Here's how the part is built. I have some questions about the finished solid (model axes, mm). Round coordinates to 2 decimals unless told otherwise and drop trailing zeros. Order: outer loops, then holes, each group sorted by start corner. A loop starts at its lowest first (then second) coordinate and runs counter-clockwise, first axis right, second up. Notation, with made-up numbers: (-18.75, 20.5) -> (-6.75, 20.5) arc R15 cw to (-6.75, 32.5) -> close; hole circle Ø2 at (74, -25). An arc over 180 degrees is marked (long way). Use a Markdown table: item, result. Add a question column.
(1) I want a section at A-A, the plane y = 12.7. Please give me the cut outline in (x, z).
(2) If I drill on probe 1 along Y at (x, z) = (0, 0.5); probe 2 along Y at (x, z) = (-12, 0.6); probe 3 along X at (y, z) = (65, 1.3), over which ranges is the centre line in solid material (lowest first)?
(3) I want a section at C-C, the plane z = 0. Please give me the cut outline in (x, y), then the cut area to 3 significant figures.
(4) I want a section at B-B, the plane x = -10. Please give me the cut outline in (y, z), then the cut area to 3 significant figures.
(5) I'm going to push flat-ended pins straight in: P1, Ø1.6, axis at x = 0.5, z = -1, coming from the +Y side; P2, Ø1, axis at y = 121.5, z = 1, coming from the -X side; P3, Ø1, axis at x = -59.5, z = 1, coming from the +Y side. Where does each tip first touch, or does it pass through?
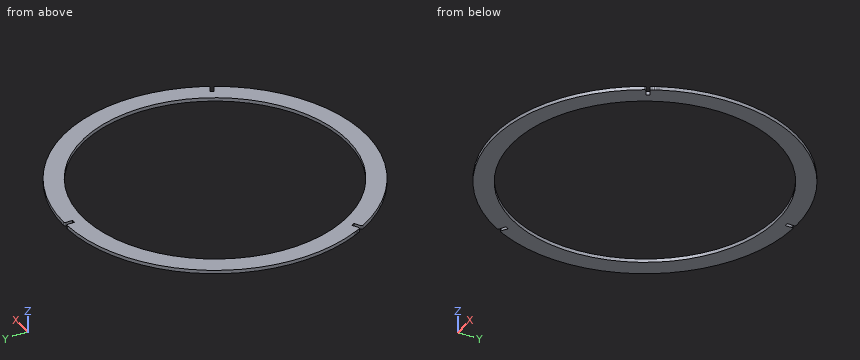
from build123d import *

# Parameters (mm, degrees)
SKETCH1_R           = 120.904
BOSS_EXTRUDE1_DEPTH = 1.5875
FILLET1_R           = 1.27


with BuildPart() as part:
    # Sketch1 → Boss-Extrude1 (new, symmetric)
    with BuildSketch(Plane.XY):
        with BuildLine():
            Line((-1.651, 142.99211797), (-1.651, 150.61211797))
            ThreePointArc((-1.651, 150.61211797), (-116.726759893, 86.166601996), (-125.058359506, -45.462572171))
            ThreePointArc((-125.058359506, -45.462572171), (-124.706816881, -46.212544567), (-124.350776736, -46.960392298))
            ThreePointArc((-124.350776736, -46.960392298), (-123.990582669, -47.705409471), (-123.625925064, -48.44825211))
            ThreePointArc((-123.625925064, -48.44825211), (-122.796227949, -50.097806374), (-121.944521887, -51.736105296))
            Line((-121.944521887, -51.736105296), (-115.42055631, -47.966631906))
            Line((-115.42055631, -47.966631906), (-113.768616335, -50.825704889))
            Line((-113.768616335, -50.825704889), (-120.366477065, -54.63787406))
            ThreePointArc((-120.366477065, -54.63787406), (-0.003414242, -125.221999958), (120.363143036, -54.643833293))
            Line((120.363143036, -54.643833293), (113.765475078, -50.831330502))
            Line((113.765475078, -50.831330502), (115.417559621, -47.972341054))
            Line((115.417559621, -47.972341054), (121.941331564, -51.742142581))
            ThreePointArc((121.941331564, -51.742142581), (122.79307438, -50.103972552), (123.622811136, -48.454547263))
            ThreePointArc((123.622811136, -48.454547263), (123.987506557, -47.711723215), (124.347738551, -46.966724405))
            ThreePointArc((124.347738551, -46.966724405), (124.703816766, -46.218894831), (125.055397569, -45.468940362))
            ThreePointArc((125.055397569, -45.468940362), (116.728630401, 86.163629972), (1.651, 150.61211797))
            Line((1.651, 150.61211797), (1.651, 142.99211797))
            Line((1.651, 142.99211797), (-1.651, 142.99211797))
        make_face()
        with Locations((0, 12.7)):
            Circle(SKETCH1_R, mode=Mode.SUBTRACT)
    extrude(amount=BOSS_EXTRUDE1_DEPTH, both=True)

    # Fillet1
    fillet1_edges = [part.edges().sort_by_distance(p)[0] for p in [
        (120.363143036, -54.643833293, 0),
        (-120.366477065, -54.63787406, 0),
        (-121.944521887, -51.736105296, 0),
        (-1.651, 150.61211797, 0),
        (1.651, 150.61211797, 0),
        (121.941331564, -51.742142581, 0),
    ]]
    fillet(fillet1_edges, radius=FILLET1_R)


solid = part.part
Taken from the geometry:
| question | item | result |
|---|---|---|
| 1 | outline | (-137.92, -1.59) -> (-120.9, -1.59) -> (-120.9, 1.59) -> (-137.92, 1.59) -> close; (120.9, -1.59) -> (137.92, -1.59) -> (137.92, 1.59) -> (120.9, 1.59) -> close |
| 2 | probe 1 | y = -125.22 to -108.2, 133.6 to 142.99 |
| 2 | probe 2 | y = -124.7 to -107.61, 133.01 to 150.1 |
| 2 | probe 3 | x = -127.62 to -109.01, 109.01 to 127.62 |
| 3 | outline | (-125.06, -45.46) arc R137.92 ccw to (-124.35, -46.96) arc R137.92 ccw to (-123.63, -48.45) arc R137.92 ccw to (-122.56, -50.56) arc R1.27 ccw to (-120.8, -51.07) -> (-115.42, -47.97) -> (-113.77, -50.83) -> (-119.28, -54.01) arc R1.27 ccw to (-119.74, -55.74) arc R137.92 ccw to (119.74, -55.74) arc R1.27 ccw to (119.27, -54.01) -> (113.77, -50.83) -> (115.42, -47.97) -> (120.79, -51.08) arc R1.27 ccw to (122.56, -50.56) arc R137.92 ccw to (124.35, -46.97) arc R137.92 ccw to (125.06, -45.47) arc R137.92 ccw to (2.95, 150.59) arc R1.27 ccw to (1.65, 149.32) -> (1.65, 142.99) -> (-1.65, 142.99) -> (-1.65, 149.32) arc R1.27 ccw to (-2.95, 150.59) arc R137.92 ccw to start; hole circle Ø241.81 at (0, 12.7) |
| 3 | area | 13,800 mm2 |
| 4 | outline | (-124.86, -1.59) -> (-107.79, -1.59) -> (-107.79, 1.59) -> (-124.86, 1.59) -> close; (133.19, -1.59) -> (150.26, -1.59) -> (150.26, 1.59) -> (133.19, 1.59) -> close |
| 4 | area | 108 mm2 |
| 5 | P1 | stops at y = 142.99 |
| 5 | P2 | stops at x = -85.4 |
| 5 | P3 | stops at y = 137.37 |
